from build123d import *

# Parameters (mm, degrees)
SKETCH1_W          = 10
SKETCH1_H          = 2
SKETCH2_R          = 1.125
CUT_EXTRUDE1_DEPTH = 15.282856857
CHAMFER2_SIZE      = 0.1


with BuildPart() as part:
    # Sketch1 → Revolve1 (revolve)
    with BuildSketch(Plane.XY, mode=Mode.PRIVATE) as revolve1_sk:
        with Locations((5, 1)):
            Rectangle(SKETCH1_W, SKETCH1_H)
    revolve(revolve1_sk.sketch.rotate(Axis((0, 0, 0), (0, 1, 0)), 90), axis=Axis((0, 0, 0), (0, 1, 0)))

    # Sketch2 → Cut-Extrude1 (cut, through all)
    with BuildSketch(Plane(origin=(0, 0, 0), x_dir=(1, 0, 0), z_dir=(0, 1, 0))):
        with Locations(Location((-1.732050808, -1, 0), (0, 0, 270))):
            Circle(SKETCH2_R)
        with Locations(Location((1.732050808, -1, 0), (0, 0, 270))):
            Circle(SKETCH2_R)
        with Locations(Location((0, 2, 0), (0, 0, 270))):
            Circle(SKETCH2_R)
    extrude(amount=CUT_EXTRUDE1_DEPTH, mode=Mode.SUBTRACT)

    # Chamfer2
    chamfer2_edges = [part.edges().sort_by_distance(p)[0] for p in [
        (0, 2, -3.125),
        (-1.732050808, 2, -0.125),
        (1.732050808, 2, -0.125),
        (0, 2, 10),
    ]]
    chamfer(chamfer2_edges, length=CHAMFER2_SIZE)


solid = part.part
The model under review builds one solid part; all positions refer to its coordinate system, in mm. Round coordinates to 2 decimals unless told otherwise and drop trailing zeros. Write each loop counter-clockwise with the first axis right and the second up, starting at its lowest first coordinate (ties: lowest second). Pieces come first, ordered by that corner, then holes. Notation, with made-up numbers: M 35.5,-20 L 64.5,-20 A10 ccw 64.5,-6 Z; hole C -33.5,-9 d7. An arc over 180 degrees is marked long. Use a Markdown table: item, result. Add a question column.
Q1. The part is to be moulded in two halves that separate along Z. For faces 1 (the face through (0, 2, 0)), 2 (the face through (0, 1, 10)), 3 (the face through (0.338, 0.937, -0.927)), say which applies: pulls with the +Z half, pulls with the -Z half, needs draft (parallel to the pull), parting line crosses it, or undercut.
Q2. To check wall thickness, follow line 1 (X direction, y = 1.4, z = 2); line 2 (X direction, y = 1.55, z = 0); line 3 (X direction, y = 0.5, z = -2) (3 decimals). State the ranges of each line that lie inside material, in increasing order.
Q3. Insertion check: pin 1 (2 mm diameter, centred on x = 5.5, z = 5.5, fed in from -Y); pin 2 (2 mm diameter, centred on x = -1.73, z = 1, fed in from +Y). Each pin has a flat end and moves straight along its axis. Give the tip position at first contact, or say it passes through.
Q4. We need section C-C, the plane y = 0.5. State the section outline as (x, z) points (3 decimals), plus the area to 3 significant figures.
Q5. We need section B-B, the plane z = 1. Count the separate pieces of the cut face and the enclosed holes in it, plus the area to 3 significant figures.
Q6. We need section A-A, the plane x = 0. State the section outline as (y, z) points (3 decimals), plus the area to 3 significant figures.
Findings below:
| question | item | result |
|---|---|---|
| 1 | face 1 | needs draft |
| 1 | face 2 | parting line crosses it |
| 1 | face 3 | undercut |
| 2 | line 1 | x = -9.8 to -2.25, -1.22 to 1.22, 2.25 to 9.8 |
| 2 | line 2 | x = -10 to -2.25, -1.22 to 1.22, 2.25 to 10 |
| 2 | line 3 | x = -9.798 to -1.125, 1.125 to 9.798 |
| 3 | pin 1 | stops at y = 0 |
| 3 | pin 2 | passes through |
| 4 | outline | C 0,0 d20; hole C -1.732,1 d2.25; hole C 0,-2 d2.25; hole C 1.732,1 d2.25 |
| 4 | area | 302 mm² |
| 5 | separate pieces | 3 |
| 5 | enclosed holes | 0 |
| 5 | area | 30.8 mm² |
| 6 | outline | M 0,-10 L 1.9,-10 L 2,-9.9 L 2,-3.225 L 1.9,-3.125 L 0,-3.125 Z; M 0,-0.875 L 1.9,-0.875 L 2,-0.775 L 2,9.9 L 1.9,10 L 0,10 Z |
| 6 | area | 35.5 mm² |
